```python
from build123d import *

# Parameters (mm, degrees)
F0_W           = 50.8
F0_H           = 25.4
F1_DEPTH       = 12.7
F3_D           = 6.35
F3_CBORE_D     = 15.24
F3_CBORE_DEPTH = 3.81
F4_R           = 3.175


with BuildPart() as f1:
    # F0 (on Top) → F1 (new body)
    with BuildSketch(Plane.XY):
        Rectangle(F0_W, F0_H)
        with BuildLine():
            Line((-25.4, -12.7), (-25.4, 12.7))
            ThreePointArc((-25.4, 12.7), (-38.1, 0), (-25.4, -12.7))
        make_face()
        with BuildLine():
            ThreePointArc((25.4, -12.7), (38.1, 0), (25.4, 12.7))
            Line((25.4, 12.7), (25.4, -12.7))
        make_face()
    extrude(amount=F1_DEPTH)

    # F3 (through all)
    with Locations(Plane.XY.offset(12.7)):
        with Locations((0, 0)):
            CounterBoreHole(F3_D / 2, F3_CBORE_D / 2, F3_CBORE_DEPTH)

    # F4
    f4_edges = [f1.edges().sort_by_distance(p)[0] for p in [
        (-38.1, 0, 12.7),
    ]]
    fillet(f4_edges, radius=F4_R)


solid = f1.part
```
For this review, take the finished solid that the model builds, in its own axes (mm). A direction names the side the tool comes from. Give positions to 0.01 mm unless a question says otherwise; leave off trailing zeros. Order: outer loops, then holes, each group sorted by start corner. A loop starts at its lowest first (then second) coordinate and runs counter-clockwise, first axis right, second up.
1) Take a section at B-B (x = 0). Give the boundary of the cut face in (y, z) (3 decimals).
2) The part is to be moulded in two halves that separate along Y. For faces 3 (the face through (0.69, -3.1, 4.38)), 4 (the face through (-38.097, 0.279, 4.696)), 5 (the face through (-0.36, 11.79, 11.75)), say which applies: released by +Y, released by -Y, zero draft, split by the parting line, or undercut.
3) Insertion check: pin 1 (10 mm diameter, centred on x = 0, y = 0, fed in from +Z); pin 2 (1 mm diameter, centred on y = -2, z = 11.5, fed in from +X); pin 3 (2 mm diameter, centred on y = -2.5, z = 4, fed in from -X). Each pin has a flat end and moves straight along its axis. Give the tip position at first contact, or say it passes through.
4) Take a section at C-C (z = 7.25). Give the boundary of the cut face in (x, y) (3 decimals), then the cut area to 3 significant figures.
5) Take a section at A-A (y = 0). Give the boundary of the cut face in (x, z) (3 decimals), then the cut area to 3 significant figures.
6) Wall thickness on line 1 (Y direction, x = 0, z = 6) (3 decimals); line 2 (Y direction, x = 0, z = 9.85); line 3 (X direction, y = 3.75, z = 10.25): over which ranges is each line inside the solid? List them lowest first.
7) For faces 1 (the face through (0, -12.7, 5)), 2 (the face through (2, -3, 8.89)), list the 3-axis set-ups (+Z, -Z, +X, -X, +Y, -Y) from which the entire face can be reached by the end or side of a thin tool; tool diameter is ignored.
Derived:
1. outline: (-12.7, 0) - (-3.175, 0) - (-3.175, 8.89) - (-7.62, 8.89) - (-7.62, 12.7) - (-9.525, 12.7) arc R3.175 ccw to (-12.7, 9.525) - close; (3.175, 0) - (12.7, 0) - (12.7, 9.525) arc R3.175 ccw to (9.525, 12.7) - (7.62, 12.7) - (7.62, 8.89) - (3.175, 8.89) - close
2. face 3: undercut
2. face 4: split by the parting line
2. face 5: released by +Y
3. pin 1: stops at z = 8.89
3. pin 2: stops at x = 37.58
3. pin 3: stops at x = -38.01
4. outline: (-25.4, -12.7) - (25.4, -12.7) arc R12.7 ccw to (25.4, 12.7) - (-25.4, 12.7) arc R12.7 ccw to start; hole circle Ø6.35 at (0, 0)
4. area: 1,770 mm2
5. outline: (-38.1, 0) - (-3.175, 0) - (-3.175, 8.89) - (-7.62, 8.89) - (-7.62, 12.7) - (-34.925, 12.7) arc R3.175 ccw to (-38.1, 9.525) - close; (3.175, 0) - (38.1, 0) - (38.1, 9.525) arc R3.175 ccw to (34.925, 12.7) - (7.62, 12.7) - (7.62, 8.89) - (3.175, 8.89) - close
5. area: 849 mm2
6. line 1: y = -12.7 to -3.175, 3.175 to 12.7
6. line 2: y = -12.68 to -7.62, 7.62 to 12.68
6. line 3: x = -37.45 to -6.63, 6.63 to 37.45
7. face 1: +Z, -Z, +X, -X, -Y
7. face 2: +Z
